For this review, take the finished solid that the model builds, in its own axes (mm). A direction names the side the tool comes from. Coordinates: 2 decimals unless noted, no trailing zeros. Order: outer loops, then holes, each group sorted by start corner. A loop starts at its lowest first (then second) coordinate and runs counter-clockwise, first axis right, second up.
from build123d import *

# Parameters (mm, degrees)
SKETCH1_R           = 3
BOSS_EXTRUDE1_DEPTH = 6
CUT_EXTRUDE1_DEPTH  = 1


with BuildPart() as part:
    # Sketch1 → Boss-Extrude1 (new body)
    with BuildSketch(Plane.XY):
        Circle(SKETCH1_R)
    extrude(amount=BOSS_EXTRUDE1_DEPTH)

    # Sketch4 → Revolve1 (revolve)
    with BuildSketch(Plane.ZY, mode=Mode.PRIVATE) as revolve1_sk:
        with BuildLine():
            Line((0, -4), (0, 0))
            Line((0, 0), (-3, 0))
            ThreePointArc((-3, 0), (-2.166666667, -2.5), (0, -4))
        make_face()
    revolve(revolve1_sk.sketch.rotate(Axis((0, 0, 0), (0, 0, -1)), 180), axis=Axis((0, 0, 0), (0, 0, -1)))

    # Sketch5 → Cut-Extrude1 (cut)
    with BuildSketch(Plane.XY.offset(-3)):
        Polygon((0, 1.811201152), (1.414213562, 0.396987589), (0.664213562, 0.396987589), (0.664213562, -1.603012411), (-0.664213562, -1.603012411), (-0.664213562, 0.396987589), (-1.414213562, 0.396987589), align=None)
    extrude(amount=CUT_EXTRUDE1_DEPTH, mode=Mode.SUBTRACT)


solid = part.part
1. Take a section at B-B, the plane x = -0.25. Give the boundary of the cut face in (y, z), plus the area to 3 significant figures.
Answer below:
outline: (-3.99, 0) arc R4.16 ccw to (-1.6, -2.67) - (-1.6, -2) - (1.56, -2) - (1.56, -2.69) arc R4.16 ccw to (3.99, 0) - (2.99, 0) - (2.99, 6) - (-2.99, 6) - (-2.99, 0) - close
area: 50.7 mm2
2. Take a section at D-D, the plane y = 2.25. Give the boundary of the cut face in (x, z), plus the area to 3 significant figures.
Answer below:
outline: (-3.31, 0) arc R3.51 ccw to (3.31, 0) - (1.98, 0) - (1.98, 6) - (-1.98, 6) - (-1.98, 0) - close
area: 35.1 mm2
3. Take a section at C-C, the plane z = 5.25. Give the boundary of the cut face in (x, y).
Answer below:
outline: circle Ø6 at (0, 0)
4. The part is to be moulded in two halves that separate along Y. For faces 3 (the face through (-3, 0, 3)), 4 (the face through (-0.664, -0.6, -2.5)), 5 (the face through (0, 0, 6)), say which applies: +Y half, -Y half, draft (parallel to the pull), parting line (faces both ways), or undercut.
Answer below:
face 3: parting line
face 4: undercut
face 5: draft
5. Machinability: for faces 1 (the face through (0.664, -0.6, -2.5)), 2 (the face through (3, 1, 0)), which of the approach directions +Z, -Z, +X, -X, +Y, -Y give a long, thin tool a straight path to every point of the face, cutting with its end or side? Answer none if there is none.
Answer below:
face 1: -Z
face 2: +Z
6. Take a section at A-A, the plane y = 0. Give the boundary of the cut face in (x, z).
Answer below:
outline: (-4, 0) arc R4.17 ccw to (-0.66, -2.95) - (-0.66, -2) - (0.66, -2) - (0.66, -2.95) arc R4.17 ccw to (4, 0) - (3, 0) - (3, 6) - (-3, 6) - (-3, 0) - close
7. To check wall thickness, follow L1, parallel to Z at x = 0.5, y = -0.25; L2, parallel to X at y = 1.25, z = 1.5; L3, parallel to Z at x = -1.75, y = 1.75. State the ranges of each line that lie inside material, in increasing order.
Answer below:
L1: z = -2 to 6
L2: x = -2.73 to 2.73
L3: z = -2.19 to 6
8. Clearance check with flat-ended pins moving along their axes: pin 1 Ø0.7 at (x, z) = (-0.5, -2.5) entering from +Y; pin 2 Ø0.6 at (x, z) = (-1, -2.5) entering from +Y; pin 3 Ø1.5 at (x, y) = (3, -3) entering from -Z. State where each tip first meets the part, or that it passes through.
Answer below:
pin 1: stops at y = 2.48
pin 2: stops at y = 2.26
pin 3: stops at z = -1.11
